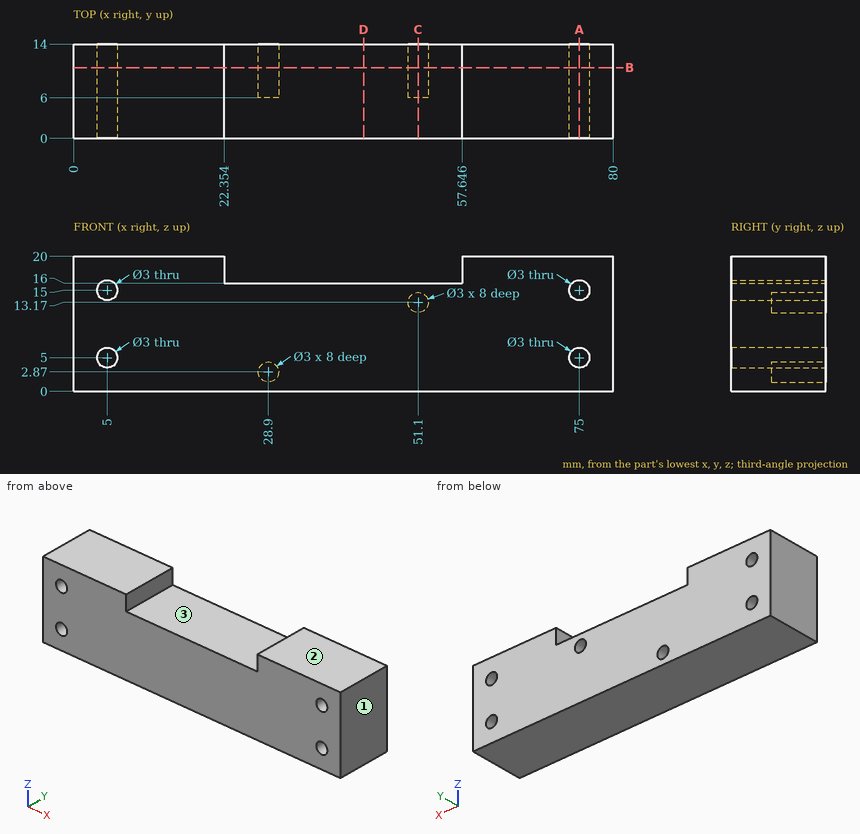
Here's the drawing with two shaded views (mm, measured from the low corner). I have some questions. Give positions to 0.01 mm unless a question says otherwise; leave off trailing zeros. Write each loop counter-clockwise with the first axis right and the second up, starting at its lowest first coordinate (ties: lowest second). Pieces come first, ordered by that corner, then holes. Notation, with made-up numbers: (-31.75, 40) -> (26.25, 40) arc R29 ccw to (26.25, 79) -> close; hole circle Ø4 at (81.25, 76.25). An arc over 180 degrees is marked (long way). Use one line per item in the form item = value.
1) Suppose I cut it at C-C (x = 51.1). Please give me the cut outline in (y, z), and give its area (3 significant figures).
Verdict:
outline = (0, 0) -> (14, 0) -> (14, 11.67) -> (6, 11.67) -> (6, 14.67) -> (14, 14.67) -> (14, 16) -> (0, 16) -> close
area = 200 mm2
2) We'd pull the mould along X, two halves only. Please class the marked faces 1, 2 and 3: +X half, -X half, draft (parallel to the pull), parting line (faces both ways), or undercut.
Verdict:
face_1 = +X half
face_2 = draft
face_3 = undercut
3) If I drill on L1, parallel to X at y = 5, z = 15; L2, parallel to Z at x = 5, y = 3.25; L3, parallel to X at y = 9.5, z = 13.17, over which ranges is the centre line in solid material (lowest first)? Write a range as [from, to].
Verdict:
L1 = [0, 3.5], [6.5, 73.5], [76.5, 80]
L2 = [0, 3.5], [6.5, 13.5], [16.5, 20]
L3 = [0, 49.6], [52.6, 80]
4) Suppose I cut it at A-A (x = 75). Please give me the cut outline in (y, z), and give its area (3 significant figures).
Verdict:
outline = (0, 0) -> (14, 0) -> (14, 3.5) -> (0, 3.5) -> close; (0, 6.5) -> (14, 6.5) -> (14, 13.5) -> (0, 13.5) -> close; (0, 16.5) -> (14, 16.5) -> (14, 20) -> (0, 20) -> close
area = 196 mm2
5) Suppose I cut it at D-D (x = 43). Please give me the cut outline in (y, z), and give its area (3 significant figures).
Verdict:
outline = (0, 0) -> (14, 0) -> (14, 16) -> (0, 16) -> close
area = 224 mm2
6) Suppose I cut it at B-B (y = 10.5). Please give me the cut outline in (x, z).
Verdict:
outline = (0, 0) -> (80, 0) -> (80, 20) -> (57.65, 20) -> (57.65, 16) -> (22.35, 16) -> (22.35, 20) -> (0, 20) -> close; hole circle Ø3 at (5, 5); hole circle Ø3 at (5, 15); hole circle Ø3 at (28.9, 2.87); hole circle Ø3 at (51.1, 13.17); hole circle Ø3 at (75, 5); hole circle Ø3 at (75, 15)
7) I'm going to push a flat-ended pin straight in: pin 1 (0.9 mm diameter, centred on x = 50.5, z = 13.5, fed in from +Y). Where does the tip first touch, or does it pass through?
Verdict:
pin_1 = 6
